Work out the finished part from the listing and answer in its coordinate system (mm). A direction names the side the tool comes from. Coordinates: 2 decimals unless noted, no trailing zeros. Write each loop counter-clockwise with the first axis right and the second up, starting at its lowest first coordinate (ties: lowest second). Pieces come first, ordered by that corner, then holes. Notation, with made-up numbers: (67, 87) - (96, 87) arc R20 cw to (96, 105) - close; hole circle Ø4 at (62, -33.5). An arc over 180 degrees is marked (long way). Use a Markdown table: item, result. Add a question column.
(1) The part is cut by section A-A, the plane y = 5. Give the vertices of the cut face in (x, z), then the cut area to 3 significant figures.
(2) Find the intervals of material crossed by line 1 (X direction, y = 9, z = -15); line 2 (Y direction, x = 0, z = -11); line 3 (X direction, y = 7, z = 0), in increasing order. Write a range as from..to.
(3) The part is cut by section B-B, the plane z = 0. Give the vertices of the cut face in (x, y), then the cut area to 4 significant figures.
(4) The part is cut by section D-D, the plane y = 14. Give the vertices of the cut face in (x, z).
(5) The part is cut by section C-C, the plane x = 38. Give the vertices of the cut face in (y, z), then the cut area to 3 significant figures.
(6) A tool of negligible diameter and unlimited length cuts with its end or side. For faces 5 (the face through (1, 6, -25)), 6 (the face through (-4, 43, 10)), 7 (the face through (-1, 12, 17)), from which of +Z, -Z, +X, -X, +Y, -Y can it reach the whole face along a straight path? Write none if from no direction.
(7) For a pull along X with two mould halves and no side action, classify faces 1 (the face through (0, 40, 11)), 2 (the face through (26, 20, -4)), 3 (the face through (3.815, 23.201, 10.612)), 4 (the face through (50, 6, 0)) as released by +X, released by -X, zero draft, split by the parting line, or undercut.
(8) Given pin 1 Ø2 at (x, z) = (30, -17.5) entering from +Y; pin 2 Ø2 at (x, z) = (-26, 1) entering from +Y; pin 3 Ø2.5 at (x, z) = (1.5, 9) entering from +Y; pin 4 Ø1 at (y, z) = (13, -19) entering from -X, each flat-ended and moving along its own axis, determine where each tip first touches the part or whether it passes through.
from build123d import *

# Parameters (mm, degrees)
SKETCH_1_R                = 4
EXTRUDE_2_DEPTH           = 12
SKETCH_4_R                = 15
SKETCH_4_R_2              = 7.5
EXTRUDE_3_DEPTH           = 33
CUT_EXTRUDE_12_DEPTH      = 84.815273071
CUT_EXTRUDE_12_DEPTH_BACK = 84.815273071
SKETCH_5_R                = 4
RIB_9_REACH               = 73.764
SKETCH_10_WALL_W          = 185.83828981
SKETCH_10_WALL_H          = 8
CUT_EXTRUDE_14_DEPTH      = 84.815273125
CUT_EXTRUDE_14_DEPTH_BACK = 84.815273125
CUT_EXTRUDE_15_DEPTH      = 72.763500535
CUT_EXTRUDE_15_DEPTH_BACK = 72.763500535
SKETCH_14_R               = 7.5


with BuildPart() as part:
    # 草图1 → 凸台-拉伸2 (new body)
    with BuildSketch(Plane(origin=(0, 0, 0), x_dir=(1, 0, 0), z_dir=(0, 1, 0))):
        with BuildLine():
            Line((-40, -25), (40, -25))
            ThreePointArc((40, -25), (47.071067812, -22.071067812), (50, -15))
            Line((50, -15), (50, 15))
            ThreePointArc((50, 15), (47.071067812, 22.071067812), (40, 25))
            Line((40, 25), (-40, 25))
            ThreePointArc((-40, 25), (-47.071067812, 22.071067812), (-50, 15))
            Line((-50, 15), (-50, -15))
            ThreePointArc((-50, -15), (-47.071067812, -22.071067812), (-40, -25))
        make_face()
        with Locations(Location((-40, 15, 0), (0, 0, 270))):
            Circle(SKETCH_1_R, mode=Mode.SUBTRACT)
        with Locations(Location((-40, -15, 0), (0, 0, 270))):
            Circle(SKETCH_1_R, mode=Mode.SUBTRACT)
        with Locations(Location((40, 15, 0), (0, 0, 270))):
            Circle(SKETCH_1_R, mode=Mode.SUBTRACT)
        with Locations(Location((40, -15, 0), (0, 0, 270))):
            Circle(SKETCH_1_R, mode=Mode.SUBTRACT)
    extrude(amount=EXTRUDE_2_DEPTH)

    # 草图4 → 凸台-拉伸3 (add)
    with BuildSketch(Plane(origin=(0, 12, 0), x_dir=(1, 0, 0), z_dir=(0, 1, 0))):
        with Locations(Location((0, 0, 0), (0, 0, 270))):
            Circle(SKETCH_4_R)
        with Locations(Location((0, 0, 0), (0, 0, 270))):
            Circle(SKETCH_4_R_2, mode=Mode.SUBTRACT)
    extrude(amount=EXTRUDE_3_DEPTH)

    # 草图5 → 切除-拉伸12 (cut, two sides: drawn at the far end of the back side and taken through both)
    with BuildSketch(Plane.XY.offset(25).offset(-CUT_EXTRUDE_12_DEPTH_BACK)):
        with Locations((0, 22)):
            Circle(SKETCH_5_R)
    extrude(amount=CUT_EXTRUDE_12_DEPTH + CUT_EXTRUDE_12_DEPTH_BACK, mode=Mode.SUBTRACT)

    # 草图10 wall → 筋9 (add, up to next)
    with BuildSketch(Plane(origin=(-32.5, 22, 0), x_dir=(0.868243142124, 0.496138938357, 0), z_dir=(-0.496138938357, 0.868243142124, 0)), mode=Mode.PRIVATE) as rib_9_sk1:
        Rectangle(SKETCH_10_WALL_W, SKETCH_10_WALL_H)
    rib_9_tool1 = extrude(rib_9_sk1.sketch, amount=-RIB_9_REACH, mode=Mode.PRIVATE) - part.part
    rib_9 = rib_9_tool1.solids().sort_by_distance((-32.5, 22, 0))[0]
    add(rib_9)

    # 草图13 → 切除-拉伸14 (cut, two sides: drawn at the far end of the back side and taken through both)
    with BuildSketch(Plane.XY.offset(25).offset(-CUT_EXTRUDE_14_DEPTH_BACK)):
        Polygon((0, 40), (4, 40), (4, 45), (0, 45), (-4, 45), (-4, 40), align=None)
    extrude(amount=CUT_EXTRUDE_14_DEPTH + CUT_EXTRUDE_14_DEPTH_BACK, mode=Mode.SUBTRACT)

    # 草图14 → 切除-拉伸15 (cut, two sides: drawn at the far end of the back side and taken through both)
    with BuildSketch(Plane(origin=(0, 0, 0), x_dir=(1, 0, 0), z_dir=(0, 1, 0)).offset(-CUT_EXTRUDE_15_DEPTH_BACK)):
        with Locations(Location((0, 0, 0), (0, 0, 122.230952636))):
            Circle(SKETCH_14_R)
    extrude(amount=CUT_EXTRUDE_15_DEPTH + CUT_EXTRUDE_15_DEPTH_BACK, mode=Mode.SUBTRACT)

    # 镜向1: 筋9 across plane
    add(rib_9.mirror(Plane(origin=(0, 0, 0), x_dir=(0, 0, 1), z_dir=(1, 0, 0))))


solid = part.part
Model answer:
| question | item | result |
|---|---|---|
| 1 | outline | (-50, -15) arc R10 ccw to (-40, -25) - (40, -25) arc R10 ccw to (50, -15) - (50, 15) arc R10 ccw to (40, 25) - (-40, 25) arc R10 ccw to (-50, 15) - close; hole circle Ø8 at (-40, -15); hole circle Ø8 at (-40, 15); hole circle Ø15 at (0, 0); hole circle Ø8 at (40, -15); hole circle Ø8 at (40, 15) |
| 1 | area | 4,540 mm^2 |
| 2 | line 1 | -50..-44, -36..36, 44..50 |
| 2 | line 2 | 0..18, 26..40 |
| 2 | line 3 | -50..-7.5, 7.5..50 |
| 3 | outline | (-50, 0) - (-7.5, 0) - (-7.5, 45) - (-15, 45) - (-15, 32) - (-50, 12) - close; (7.5, 0) - (50, 0) - (50, 12) - (15, 32) - (15, 45) - (7.5, 45) - close |
| 3 | area | 2,215 mm^2 |
| 4 | outline | (-46.5, -4) - (-14.46, -4) arc R15 ccw to (14.46, -4) - (46.5, -4) - (46.5, 4) - (14.46, 4) arc R15 ccw to (-14.46, 4) - (-46.5, 4) - close; hole circle Ø15 at (0, 0) |
| 5 | outline | (0, -25) - (12, -25) - (12, -18.46) - (0, -18.46) - close; (0, -11.54) - (12, -11.54) - (12, -4) - (18.86, -4) - (18.86, 4) - (12, 4) - (12, 11.54) - (0, 11.54) - close; (0, 18.46) - (12, 18.46) - (12, 25) - (0, 25) - close |
| 5 | area | 489 mm^2 |
| 6 | face 5 | -Z, +X, -X, +Y, -Y |
| 6 | face 6 | +Z, -Z, +Y |
| 6 | face 7 | +Z, +Y |
| 7 | face 1 | undercut |
| 7 | face 2 | zero draft |
| 7 | face 3 | undercut |
| 7 | face 4 | released by +X |
| 8 | pin 1 | y = 12 |
| 8 | pin 2 | y = 26.29 |
| 8 | pin 3 | y = 40 |
| 8 | pin 4 | through |
